Geometry check sheet. Reference: drawing and pictorial views, mm from the part's lowest x, y, z. A direction names the side the tool comes from. Round coordinates to 2 decimals unless told otherwise and drop trailing zeros. Order: outer loops, then holes, each group sorted by start corner. A loop starts at its lowest first (then second) coordinate and runs counter-clockwise, first axis right, second up.
Q1. Cross-section at D-D on y = 6.5. Record the cut outline in (x, z).
Q2. Scan lines: probe 1 along Y at (x, z) = (21, 24.5); probe 2 along Z at (x, y) = (19, 28.5); probe 3 along Z at (x, y) = (20, 6). Record each from-to range of solid material in increasing order.
Q3. Cross-section at A-A on y = 21. Record the cut outline in (x, z), then the cut area to 3 significant figures.
Q4. Set-up check for the marked faces 1 and 2: record each of +Z, -Z, +X, -X, +Y, -Y from which the full face is reachable in a straight line by a thin tool's end or side.
Q5. Depth check by flat-ended pin: P1, Ø7, axis at x = 21, y = 18, coming from the -Z side; P2, Ø10, axis at x = 8, z = 40.5, coming from the +Y side; P3, Ø2, axis at x = 14, z = 15, coming from the -Y side. Enter the tip coordinate at first touch or a pass-through.
Q6. Mould release check, pull along Y, two halves, no side actions. Record for the marked faces 3, 4 and 5: +Y half, -Y half, draft (parallel to the pull), parting line (faces both ways), or undercut.
Q7. Cross-section at C-C on z = 66.5. Record the cut outline in (x, y).
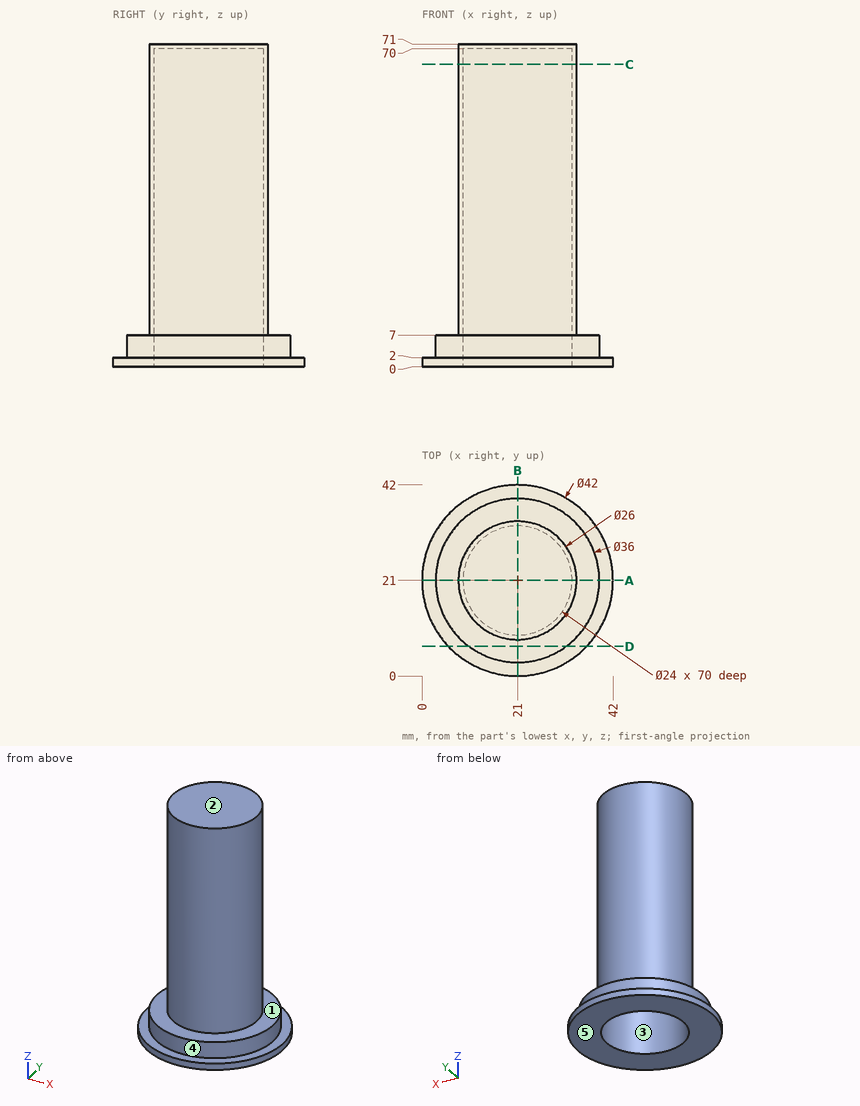
Results found:
1. outline: (5.81, 0) - (36.19, 0) - (36.19, 2) - (31.67, 2) - (31.67, 7) - (10.33, 7) - (10.33, 2) - (5.81, 2) - close
2. probe 1: y = 8 to 9, 33 to 34
2. probe 2: z = 70 to 71
2. probe 3: z = 0 to 7
3. outline: (0, 0) - (9, 0) - (9, 70) - (33, 70) - (33, 0) - (42, 0) - (42, 2) - (39, 2) - (39, 7) - (34, 7) - (34, 71) - (8, 71) - (8, 7) - (3, 7) - (3, 2) - (0, 2) - close
3. area: 248 mm2
4. face 1: +Z
4. face 2: +Z, +X, -X, +Y, -Y
5. P1: stops at z = 70
5. P2: stops at y = 31.25
5. P3: stops at y = 9.47
6. face 3: undercut
6. face 4: parting line
6. face 5: draft
7. outline: circle Ø26 at (21, 21); hole circle Ø24 at (21, 21)
